Autodesk Inventor part; units mm, degrees
ref_plane "YZ Plane" through (0, 0, 0) normal (1, 0, 0) x (0, 1, 0)
ref_plane "XZ Plane" through (0, 0, 0) normal (0, 1, 0) x (-1, 0, 0)
ref_plane "XY Plane" through (0, 0, 0) normal (0, 0, 1) x (1, 0, 0)
sketch "Эскиз1" plane through (0, 0, 0) normal (0, 0, 1) x (1, 0, 0)
  circle A0 centre (0, 0) radius 62
  circle A1 centre (0, 0) radius 22.5
  dimension "d0" = 124
  dimension "d15" = 45
extrude "Выдавливание1" add sketch "Эскиз1" along normal blind 2
sketch "Эскиз2" plane through (0, 0, 2) normal (0, 0, 1) x (1, 0, 0)
  arc A0 (17, 29.4449) -> (-17, 29.4449) centre (0, 0) ccw construction
  arc A1 (19, 32.909) -> (-19, 32.909) centre (0, 0) ccw
  arc A2 (15, 25.9808) -> (-15, 25.9808) centre (0, 0) ccw
  arc A3 (15, 25.9808) -> (19, 32.909) centre (17, 29.4449) ccw
  arc A4 (-19, 32.909) -> (-15, 25.9808) centre (-17, 29.4449) ccw
  line L0 (0, 0) -> (-17, 29.4449) construction
  line L1 (0, 0) -> (34, 0) construction
  line L2 (0, 0) -> (17, 29.4449) construction
  arc A5 (25, 43.3013) -> (-25, 43.3013) centre (0, 0) ccw construction
  arc A6 (27, 46.7654) -> (-27, 46.7654) centre (0, 0) ccw
  arc A7 (23, 39.8372) -> (-23, 39.8372) centre (0, 0) ccw
  arc A8 (23, 39.8372) -> (27, 46.7654) centre (25, 43.3013) ccw
  arc A9 (-27, 46.7654) -> (-23, 39.8372) centre (-25, 43.3013) ccw
  line L3 (0, 0) -> (-25, 43.3013) construction
  line L4 (0, 0) -> (50, 0) construction
  line L5 (0, 0) -> (25, 43.3013) construction
  arc A10 (33, 57.1577) -> (-33, 57.1577) centre (0, 0) ccw construction
  line L6 (0, 0) -> (-33, 57.1577) construction
  line L7 (0, 0) -> (66, 0) construction
  line L8 (0, 0) -> (33, 57.1577) construction
  dimension "d3" = 34
  dimension "d4" = 120
  dimension "d5" = 60
  dimension "d6" = 8
  dimension "d7" = 50
  dimension "d8" = 120
  dimension "d9" = 60
  dimension "d10" = 8
  dimension "d11" = 66
  dimension "d12" = 120
  dimension "d13" = 60
extrude "Выдавливание2" cut sketch "Эскиз2" against normal through all
pattern_circular "Круговой массив1" count 3 over 360 about axis through (0, 0, 0) along (0, 0, 1) of "Выдавливание2"
properties part number "Ограничитель" material "Сталь, высокопрочная, низколегированная"
The listing builds one solid part. Answer for the finished solid, in the listing's coordinates (mm). A direction names the side the tool comes from. Round coordinates to 2 decimals unless told otherwise and drop trailing zeros. Write each loop counter-clockwise with the first axis right and the second up, starting at its lowest first coordinate (ties: lowest second). Pieces come first, ordered by that corner, then holes. Notation, with made-up numbers: (33.5, 2) -> (87.5, 2) arc R8 ccw to (87.5, 15) -> close; hole circle Ø11 at (64, 34). An arc over 180 degrees is marked (long way). Use CSV: the item, a comma, the result in double quotes. Start each with the question number.
(1) Section B-B on y = 19 is taken. Give the vertices of the cut face in (x, z).
(2) Section C-C on x = 51.5 is taken. Give the vertices of the cut face in (y, z), then the cut area to 3 significant figures.
(3) Section D-D on z = 1 is taken. Give the vertices of the cut face in (x, y).
(4) Consider L1, parallel to Y at x = 0, z = 0.9; L2, parallel to X at y = -13.5, z = 0.2; L3, parallel to Y at x = 6.5, z = 1.35. Determine where each line is inside the solid, lowest interval first. Write a range as from..to.
(5) Which of the six approach directions +Z, -Z, +X, -X, +Y, -Y give full straight-line access (tool end or side, diameter ignored) to faces 1 (the face through (50, 4, 1)), 2 (the face through (27, 1, 0))?
(6) Section A-A on x = 0 is taken. Give the vertices of the cut face in (y, z).
(7) The mould has two halves that part along X. Classify faces 3 (the face through (25.87, -15.19, 1.01)), 4 (the face through (-8.071, -61.472, 0.986)), 5 (the face through (27, 1, 2)): released by +X, released by -X, zero draft, split by the parting line, or undercut.
(8) This flat-tipped pin is pushed along its axis until it touches: pin 1 (1 mm diameter, centred on x = 37, z = 1, fed in from -Y). Where does it stop, or does it pass through?
A:
1,outline,"(-59.02, 0) -> (-12.05, 0) -> (-12.05, 2) -> (-59.02, 2) -> close; (12.05, 0) -> (59.02, 0) -> (59.02, 2) -> (12.05, 2) -> close"
2,outline,"(-34.52, 0) -> (-16.24, 0) -> (-16.24, 2) -> (-34.52, 2) -> close; (3.71, 0) -> (34.52, 0) -> (34.52, 2) -> (3.71, 2) -> close"
2,area,"98.2 mm²"
3,outline,"circle Ø124 at (0, 0); hole (-54, 0) arc R54 ccw to (-27, -46.77) arc R4 ccw to (-23, -39.84) arc R46 cw to (-46, 0) arc R4 ccw to start; hole (-38, 0) arc R38 ccw to (-19, -32.91) arc R4 ccw to (-15, -25.98) arc R30 cw to (-30, 0) arc R4 ccw to start; hole (-27, 46.77) arc R4 ccw to (-23, 39.84) arc R46 cw to (23, 39.84) arc R4 ccw to (27, 46.77) arc R54 ccw to start; hole circle Ø45 at (0, 0); hole (-19, 32.91) arc R4 ccw to (-15, 25.98) arc R30 cw to (15, 25.98) arc R4 ccw to (19, 32.91) arc R38 ccw to start; hole (15, -25.98) arc R4 ccw to (19, -32.91) arc R38 ccw to (38, 0) arc R4 ccw to (30, 0) arc R30 cw to start; hole (23, -39.84) arc R4 ccw to (27, -46.77) arc R54 ccw to (54, 0) arc R4 ccw to (46, 0) arc R46 cw to start"
4,L1,"y = -62..-22.5, 22.5..30, 38..46, 54..62"
4,L2,"x = -60.51..-52.29, -43.97..-35.52, -26.79..-18, 18..26.79, 35.52..43.97, 52.29..60.51"
4,L3,"y = -61.66..-21.54, 21.54..29.29, 37.44..45.54, 53.61..61.66"
5,face 1,"+Z, -Z"
5,face 2,"-Z, +X, -X, +Y, -Y"
6,outline,"(-62, 0) -> (-22.5, 0) -> (-22.5, 2) -> (-62, 2) -> close; (22.5, 0) -> (30, 0) -> (30, 2) -> (22.5, 2) -> close; (38, 0) -> (46, 0) -> (46, 2) -> (38, 2) -> close; (54, 0) -> (62, 0) -> (62, 2) -> (54, 2) -> close"
7,face 3,"undercut"
7,face 4,"split by the parting line"
7,face 5,"zero draft"
8,pin 1,"stops at y = -50.12"
